Can you work these out from the model? Positions are in its coordinate system, mm. A direction names the side the tool comes from. Give positions to 0.01 mm unless a question says otherwise; leave off trailing zeros. Order: outer loops, then holes, each group sorted by start corner. A loop starts at its lowest first (then second) coordinate and runs counter-clockwise, first axis right, second up. Notation, with made-up numbers: (-18.5, 47.25) - (33.5, 47.25) arc R18 ccw to (33.5, 55.25) - close; hole circle Ø1 at (-18, -16.5). An arc over 180 degrees is marked (long way). Answer as a JSON object with one key per item and string values.
```python
from build123d import *

# Parameters (mm, degrees)
SKETCH_1_R          = 32.5
SKETCH_1_R_2        = 20
EXTRUDE_3_REACH     = 102.5
SKETCH_5_R          = 25
SKETCH_9_R          = 16
CUT_EXTRUDE_3_DEPTH = 80


with BuildPart() as part:
    # 扫描1: sweep along a path in 草图2
    with BuildLine(Plane.XY) as sweep_1_path:
        ThreePointArc((0, 0), (-19.916738879, 48.083261121), (-68, 68))
    # 草图1 → 扫描1 (sweep)
    with BuildSketch(Plane(origin=(0, 0, 0), x_dir=(1, 0, 0), z_dir=(0, 1, 0))):
        Circle(SKETCH_1_R)
        Circle(SKETCH_1_R_2, mode=Mode.SUBTRACT)
    sweep(path=sweep_1_path.line)

    # 草图5 → 凸台-拉伸3 (add, up to next)
    with BuildSketch(Plane(origin=(0, 100.5, 0), x_dir=(1, 0, 0), z_dir=(0, 1, 0)), mode=Mode.PRIVATE) as extrude_3_sk1:
        with Locations((-8, 0)):
            Circle(SKETCH_5_R)
    extrude_3_tool1 = extrude(extrude_3_sk1.sketch, amount=-EXTRUDE_3_REACH, mode=Mode.PRIVATE) - part.part
    add(extrude_3_tool1.solids().sort_by_distance((-8, 100.5, 0))[0])

    # 草图9 → 切除-拉伸3 (cut)
    with BuildSketch(Plane(origin=(0, 100.5, 0), x_dir=(1, 0, 0), z_dir=(0, 1, 0))):
        with Locations((-8, 0)):
            Circle(SKETCH_9_R)
    extrude(amount=-CUT_EXTRUDE_3_DEPTH, mode=Mode.SUBTRACT)


solid = part.part
```
Q1. We'd pull the mould along X, two halves only. Please class faces 3 (the face through (-68, 83, -14)), 4 (the face through (14, 0, -15)), 5 (the face through (6.78, 79.06, 6.13)): released by +X, released by -X, zero draft, split by the parting line, or undercut.
Recorded:
{"face 3": "released by -X", "face 4": "zero draft", "face 5": "undercut"}
Q2. Which directions (+Z, -Z, +X, -X, +Y, -Y) give clear straight access to the entire face, cutting with the end or side of a thin tool? Please do faces 1 (the face through (15.846, 82.598, -7.509)), 2 (the face through (-8.3, 100.5, 16.3)).
Recorded:
{"face 1": "+Y", "face 2": "+Z, -Z, +X, -X, +Y"}
Q3. I need wall thicknesses on L1, parallel to Z at x = -8, y = 81; L2, parallel to Y at x = -59, z = 12.5; L3, parallel to Z at x = -6, y = 64.5. Which ranges of each line are inside material? Lowest first, please.
Recorded:
{"L1": "z = -25 to -16, 16 to 25", "L2": "y = 36.92 to 51.61, 83.13 to 97.59", "L3": "z = -24.92 to -15.87, 15.87 to 24.92"}
Q4. If we section it at B-B, the plane z = 7: Please give me the cut outline in (x, y) (1 decimal), then the cut area to 3 significant figures.
Recorded:
{"outline": "(-68, 36.3) arc R36.3 cw to (-31.7, 0) - (-18.7, 0) arc R49.3 ccw to (-68, 49.3) - close; (-68, 86.7) arc R86.7 cw to (-22.4, 73.8) - (-22.4, 100.5) - (-32, 100.5) - (-32, 93) arc R99.7 ccw to (-68, 99.7) - close; (6.4, 44.6) arc R86.7 cw to (18.7, 0) - (31.7, 0) arc R99.7 ccw to (16, 53.8) - (16, 100.5) - (6.4, 100.5) - close", "area": "2,750 mm^2"}
Q5. I'm going to push flat-ended pins straight in: pin 1 Ø4 at (y, z) = (42, 13) entering from +X; pin 2 Ø1 at (x, z) = (-1, -14.5) entering from -Y (3 decimals); pin 3 Ø12 at (x, y) = (6.5, 11) entering from +Z. Where does each tip first touch, or does it pass through?
Recorded:
{"pin 1": "stops at x = 21.6", "pin 2": "stops at y = 45.685", "pin 3": "stops at z = 32.47"}
Q6. If we section it at A-A, the plane z = -9: Please give me the cut outline in (x, y).
Recorded:
{"outline": "(-68, 36.77) arc R36.77 cw to (-31.23, 0) - (-17.86, 0) arc R50.14 ccw to (-68, 50.14) - close; (-68, 85.86) arc R85.86 cw to (-21.23, 72) - (-21.23, 100.5) - (-31.32, 100.5) - (-31.32, 92.2) arc R99.23 ccw to (-68, 99.23) - close; (5.23, 44.83) arc R85.86 cw to (17.86, 0) - (31.23, 0) arc R99.23 ccw to (15.32, 53.88) - (15.32, 100.5) - (5.23, 100.5) - close"}
